Source: CAD feature listing. Evaluate the final solid. Frame: model axes, mm. Face numbers are marked on the shaded views. Round coordinates to 2 decimals unless told otherwise and drop trailing zeros. Order: outer loops, then holes, each group sorted by start corner. A loop starts at its lowest first (then second) coordinate and runs counter-clockwise, first axis right, second up. Notation, with made-up numbers: M 44,45 L 71,45 A21 cw 71,65 Z; hole C 35,-8 d6. An arc over 180 degrees is marked long. Use CSV: the item, a comma, the result in double quotes. Start each with the question number.
```python
from build123d import *

# Parameters (mm, degrees)
SKETCH1_W                = 38
SKETCH1_H                = 10
BOSS_EXTRUDE1_DEPTH      = 3
SKETCH2_R                = 2.472864358
SKETCH2_R_2              = 1
CUT_EXTRUDE1_DEPTH       = 3
FILLET1_R                = 3
F_3_0_3_DIAMETER_HOLE1_D = 3


with BuildPart() as part:
    # Sketch1 → Boss-Extrude1 (new body)
    with BuildSketch(Plane(origin=(0, 0, 0), x_dir=(1, 0, 0), z_dir=(0, 1, 0))):
        Rectangle(SKETCH1_W, SKETCH1_H)
    extrude(amount=BOSS_EXTRUDE1_DEPTH)

    # Sketch2 → Cut-Extrude1 (cut)
    with BuildSketch(Plane(origin=(0, 3, 0), x_dir=(1, 0, 0), z_dir=(0, 1, 0))):
        with Locations((15, 0)):
            Circle(SKETCH2_R)
        with Locations((6.55, 0)):
            Circle(SKETCH2_R_2)
        with Locations((2.55, 0)):
            Circle(SKETCH2_R_2)
    extrude(amount=-CUT_EXTRUDE1_DEPTH, mode=Mode.SUBTRACT)

    # Fillet1
    fillet1_edges = [part.edges().sort_by_distance(p)[0] for p in [
        (19, 1.5, 5),
        (-19, 1.5, 5),
        (-19, 1.5, -5),
        (19, 1.5, -5),
    ]]
    fillet(fillet1_edges, radius=FILLET1_R)

    # Ø3.0 (3) Diameter Hole1 (through all)
    with Locations(Plane(origin=(0, 3, 0), x_dir=(1, 0, 0), z_dir=(0, 1, 0))):
        with Locations((-15, 0)):
            Hole(F_3_0_3_DIAMETER_HOLE1_D / 2)


solid = part.part
```
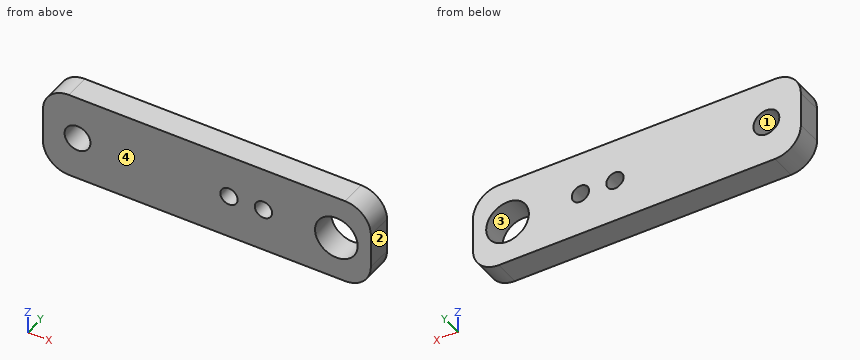
(1) Section D-D on x = 15. Return loops of the section in (y, z).
(2) Draft query along X for the marked faces 1, 2, 3 and 4. Return one class per face: pulls with the +X half, pulls with the -X half, needs draft (parallel to the pull), parting line crosses it, or undercut.
(3) Section B-B on z = 0. Return loops of the section in (x, y).
(4) Section A-A on x = 2.55. Return loops of the section in (y, z).
(5) Line query: line 1 along Z through (x, y) = (2.55, 1.05); line 2 along X through (y, z) = (0.6, -0.75); line 3 along X through (y, z) = (0.6, 1.75). Output: solid intervals per line, ascending.
(6) Section C-C on y = 1.7. Return loops of the section in (x, z).
Results below:
1,outline,"M 0,-5 L 3,-5 L 3,-2.47 L 0,-2.47 Z; M 0,2.47 L 3,2.47 L 3,5 L 0,5 Z"
2,face 1,"undercut"
2,face 2,"pulls with the +X half"
2,face 3,"undercut"
2,face 4,"needs draft"
3,outline,"M -19,0 L -16.5,0 L -16.5,3 L -19,3 Z; M -13.5,0 L 1.55,0 L 1.55,3 L -13.5,3 Z; M 3.55,0 L 5.55,0 L 5.55,3 L 3.55,3 Z; M 7.55,0 L 12.53,0 L 12.53,3 L 7.55,3 Z; M 17.47,0 L 19,0 L 19,3 L 17.47,3 Z"
4,outline,"M 0,-5 L 3,-5 L 3,-1 L 0,-1 Z; M 0,1 L 3,1 L 3,5 L 0,5 Z"
5,line 1,"z = -5 to -1, 1 to 5"
5,line 2,"x = -19 to -16.3, -13.7 to 1.89, 3.21 to 5.89, 7.21 to 12.64, 17.36 to 19"
5,line 3,"x = -19 to 13.25, 16.75 to 19"
6,outline,"M -19,-2 A3 ccw -16,-5 L 16,-5 A3 ccw 19,-2 L 19,2 A3 ccw 16,5 L -16,5 A3 ccw -19,2 Z; hole C -15,0 d3; hole C 2.55,0 d2; hole C 6.55,0 d2; hole C 15,0 d4.95"
